The listing builds one solid part. Answer for the finished solid, in the listing's coordinates (mm). Face numbers are marked on the shaded views. A direction names the side the tool comes from. Give positions to 0.01 mm unless a question says otherwise; leave off trailing zeros. Loops run counter-clockwise (first coordinate to the right, second up) from the corner with the lowest first, then second, coordinate; pieces in that order, holes last.
Item 1: Section D-D, the plane x = -58.75 is taken. Give the vertices of the cut face in (y, z), and give its area (3 significant figures).
Item 2: The mould has two halves that part along X. Classify the marked faces 1, 2 and 3: pulls with the +X half, pulls with the -X half, needs draft (parallel to the pull), parting line crosses it, or undercut.
Item 3: A tool of negligible diameter and unlimited length cuts with its end or side. For the marked faces 4, 5 and 6, from which of +Z, -Z, +X, -X, +Y, -Y can it reach the whole face along a straight path? Write none if from no direction.
Item 4: Section B-B, the plane y = -2110.5 is taken. Give the vertices of the cut face in (x, z).
Item 5: Consider line 1 along Z through (x, y) = (-54, -2110.5); line 2 along Z through (x, y) = (-54.75, -2110.5); line 3 along X through (y, z) = (-2105.5, -184). Determine where each line is inside the solid, lowest interval first.
Item 6: Section C-C, the plane z = -181.5 is taken. Give the vertices of the cut face in (x, y), and give its area (3 significant figures).
Item 7: Section A-A, the plane z = -162 is taken. Give the vertices of the cut face in (x, y), and give its area (3 significant figures).
Item 8: Each of these flat-tipped pins is pushed along its axis until it touches: pin 1 Ø4 at (x, y) = (-44.55, -2106.39) entering from +Z; pin 2 Ø1.8 at (x, z) = (-53.5, -174) entering from -Y; pin 3 Ø1 at (y, z) = (-2107, -178) entering from -X. Where does it stop, or does it pass through?
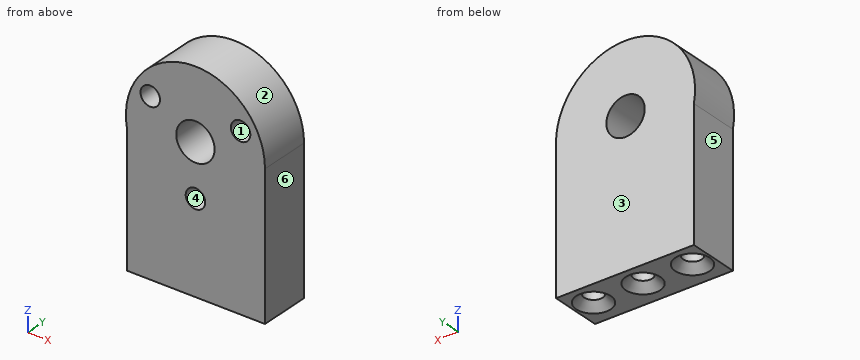
from build123d import *

# Parameters (mm, degrees)
SKETCH2_R                                      = 12.7
BOSS_EXTRUDE6_DEPTH                            = 40.64
SKETCH3_R                                      = 3.5
CUT_EXTRUDE1_DEPTH                             = 40.64
SKETCH4_R                                      = 1.778
CUT_EXTRUDE2_DEPTH                             = 6
BOSS_EXTRUDE8_DEPTH                            = 10
SKETCH8_W                                      = 25.185693912
SKETCH8_H                                      = 10
BOSS_EXTRUDE9_DEPTH                            = 7.284789
BOSS_EXTRUDE10_DEPTH                           = 30.64
CSK_FOR_M3_FLAT_HEAD_MACHINE_SCREW1_AT_2_COUNT = 2
CSK_FOR_M3_FLAT_HEAD_MACHINE_SCREW1_AT_2_PITCH = 9.039543014
CSK_FOR_M3_FLAT_HEAD_MACHINE_SCREW1_AT_3_COUNT = 2
CSK_FOR_M3_FLAT_HEAD_MACHINE_SCREW1_AT_3_PITCH = 9.039543014
SKETCH25_W                                     = 26.719153215
SKETCH25_H                                     = 31.319175306
CUT_EXTRUDE9_DEPTH                             = 39.778747573


with BuildPart() as part:
    # Sketch2 → Boss-Extrude6 (new body)
    with BuildSketch(Plane(origin=(0, -2111.389926236, 0), x_dir=(1, 0, 0), z_dir=(0, 1, 0))):
        with Locations((-53.693967541, 163.840329354)):
            Circle(SKETCH2_R)
    extrude(amount=BOSS_EXTRUDE6_DEPTH)

    # Sketch3 → Cut-Extrude1 (cut)
    with BuildSketch(Plane(origin=(0, -2070.749926236, 0), x_dir=(1, 0, 0), z_dir=(0, 1, 0))):
        with Locations((-53.693967541, 163.840329354)):
            Circle(SKETCH3_R)
    extrude(amount=-CUT_EXTRUDE1_DEPTH, mode=Mode.SUBTRACT)

    # Sketch4 → Cut-Extrude2 (cut)
    with BuildSketch(Plane.XZ.offset(2111.389926236)):
        with Locations((-61.942859512, -159.077829354)):
            Circle(SKETCH4_R)
        with Locations((-53.693967541, -173.365329354)):
            Circle(SKETCH4_R)
        with Locations((-45.44507557, -159.077829354)):
            Circle(SKETCH4_R)
    extrude(amount=-CUT_EXTRUDE2_DEPTH, mode=Mode.SUBTRACT)

    # Sketch7 → Boss-Extrude8 (add)
    with BuildSketch(Plane.XZ.offset(2111.389926236)):
        with BuildLine():
            Line((-40.993967541, -163.840329354), (-40.993967541, -182.634287878))
            Line((-40.993967541, -182.634287878), (-66.179661453, -182.634287878))
            Line((-66.179661453, -182.634287878), (-66.179661453, -166.163570095))
            ThreePointArc((-66.179661453, -166.163570095), (-52.527415502, -176.486639343), (-40.993967541, -163.840329354))
        make_face()
    extrude(amount=-BOSS_EXTRUDE8_DEPTH)

    # Sketch8 → Boss-Extrude9 (add)
    with BuildSketch(Plane(origin=(0, 0, -182.634287878), x_dir=(-1, 0, 0), z_dir=(0, 0, -1))):
        with Locations((53.586814497, -2106.389926236)):
            Rectangle(SKETCH8_W, SKETCH8_H)
    extrude(amount=BOSS_EXTRUDE9_DEPTH)

    # Sketch9 → Boss-Extrude10 (add)
    with BuildSketch(Plane(origin=(0, -2070.749926236, 0), x_dir=(1, 0, 0), z_dir=(0, 1, 0))):
        with BuildLine():
            Line((-66.179661453, 163.840329354), (-66.179661453, 189.919076927))
            Line((-66.179661453, 189.919076927), (-40.993967541, 189.919076927))
            Line((-40.993967541, 189.919076927), (-40.993967541, 163.840329354))
            ThreePointArc((-40.993967541, 163.840329354), (-53.586814497, 176.43317631), (-66.179661453, 163.840329354))
        make_face()
    extrude(amount=-BOSS_EXTRUDE10_DEPTH)

    # Sketch15 → CSK for M3 Flat Head Machine Screw1 (revolve, cut)
    with BuildSketch(Plane(origin=(-53.586814498, -2075.749926236, -189.919076927), x_dir=(0, 1, 0), z_dir=(1, 0, 0))):
        Polygon((0, 0), (0, 10), (1.7, 8.978536948), (1.7, 1.45), (3.15, 0), align=None)
    csk_for_m3_flat_head_machine_screw1 = revolve(axis=Axis((-53.586814498, -2075.749926236, -196.269076927), (0, 0, 1)), mode=Mode.SUBTRACT)

    # CSK for M3 Flat Head Machine Screw1 at 2: CSK for M3 Flat Head Machine Screw1 ×2
    with Locations(*[(-i * CSK_FOR_M3_FLAT_HEAD_MACHINE_SCREW1_AT_2_PITCH, 0, 0) for i in range(1, CSK_FOR_M3_FLAT_HEAD_MACHINE_SCREW1_AT_2_COUNT)]):
        add(csk_for_m3_flat_head_machine_screw1, mode=Mode.SUBTRACT)

    # CSK for M3 Flat Head Machine Screw1 at 3: CSK for M3 Flat Head Machine Screw1 ×2
    with Locations(*[(i * CSK_FOR_M3_FLAT_HEAD_MACHINE_SCREW1_AT_3_PITCH, 0, 0) for i in range(1, CSK_FOR_M3_FLAT_HEAD_MACHINE_SCREW1_AT_3_COUNT)]):
        add(csk_for_m3_flat_head_machine_screw1, mode=Mode.SUBTRACT)

    # Mirror1: CSK for M3 Flat Head Machine Screw1 across plane
    add(csk_for_m3_flat_head_machine_screw1.mirror(Plane.ZX.offset(-2091.069926234)), mode=Mode.SUBTRACT)

    # Mirror1 copy 1 sketch → Mirror1 copy 1 (revolve, cut)
    with BuildSketch(Plane(origin=(-62.626357512, -2106.389926232, -189.919076927), x_dir=(0, -1, 0), z_dir=(1, 0, 0))):
        Polygon((0, 0), (0, -10), (1.7, -8.978536948), (1.7, -1.45), (3.15, 0), align=None)
    revolve(axis=Axis((-62.626357512, -2106.389926232, -196.269076927), (0, 0, -1)), mode=Mode.SUBTRACT)

    # Mirror1 copy 2 sketch → Mirror1 copy 2 (revolve, cut)
    with BuildSketch(Plane(origin=(-44.547271484, -2106.389926232, -189.919076927), x_dir=(0, -1, 0), z_dir=(1, 0, 0))):
        Polygon((0, 0), (0, -10), (1.7, -8.978536948), (1.7, -1.45), (3.15, 0), align=None)
    revolve(axis=Axis((-44.547271484, -2106.389926232, -196.269076927), (0, 0, -1)), mode=Mode.SUBTRACT)

    # Sketch25 → Cut-Extrude9 (cut, through all)
    with BuildSketch(Plane(origin=(0, 0, -189.919076927), x_dir=(-1, 0, 0), z_dir=(0, 0, -1))):
        with Locations((54.353544149, -2086.409513889)):
            Rectangle(SKETCH25_W, SKETCH25_H)
    extrude(amount=-CUT_EXTRUDE9_DEPTH, mode=Mode.SUBTRACT)


solid = part.part
Worked answers:
1. outline: (-2111.39, -189.92) - (-2102.07, -189.92) - (-2102.07, -152.19) - (-2111.39, -152.19) - close
1. area: 352 mm2
2. face 1: undercut
2. face 2: parting line crosses it
2. face 3: needs draft
3. face 4: -Y
3. face 5: -Z, -X, +Y, -Y
3. face 6: +Z, -Z, +X, +Y, -Y
4. outline: (-66.18, -189.92) - (-40.99, -189.92) - (-40.99, -163.84) arc R12.7 ccw (long way) to (-66.18, -166.16) - close; hole circle Ø3.56 at (-61.94, -159.08); hole circle Ø7 at (-53.69, -163.84); hole circle Ø3.56 at (-53.69, -173.37); hole circle Ø3.56 at (-45.45, -159.08)
5. line 1: z = -189.92 to -175.12, -171.61 to -167.33, -160.35 to -151.14
5. line 2: z = -189.92 to -174.8, -171.93 to -167.18, -160.5 to -151.18
5. line 3: x = -66.18 to -64.07, -61.18 to -55.04, -52.14 to -46, -43.1 to -40.99
6. outline: (-66.18, -2111.39) - (-40.99, -2111.39) - (-40.99, -2102.07) - (-66.18, -2102.07) - close; hole circle Ø3.4 at (-62.63, -2106.39); hole circle Ø3.4 at (-53.59, -2106.39); hole circle Ø3.4 at (-44.55, -2106.39)
6. area: 208 mm2
7. outline: (-66.26, -2111.39) - (-56.67, -2111.39) - (-56.67, -2102.07) - (-66.26, -2102.07) - close; (-50.72, -2111.39) - (-41.13, -2111.39) - (-41.13, -2102.07) - (-50.72, -2102.07) - close
7. area: 179 mm2
8. pin 1: stops at z = -153.34
8. pin 2: stops at y = -2105.39
8. pin 3: stops at x = -66.18
